from build123d import *

# Parameters (mm, degrees)
F0_R     = 6.477
F1_DEPTH = 6.35
F0_W     = 6.35
F0_H     = 25.4
F2_DEPTH = 6.35
F3_DEPTH = 6.35
F4_DEPTH = 6.35
F5_DEPTH = 6.35


with BuildPart() as f1:
    # F0 (on Top) → F1 (new body)
    with BuildSketch(Plane.XY):
        Polygon((184.15, 76.2), (-184.15, 76.2), (-184.15, 50.8), (-184.15, 25.4), (-184.15, 0), (-184.15, -25.4), (-184.15, -50.8), (-184.15, -76.2), (184.15, -76.2), (184.15, -50.8), (184.15, -25.4), (184.15, 0), (184.15, 25.4), (184.15, 50.8), align=None)
        with BuildLine():
            ThreePointArc((-157.1244, 0), (-163.6014, -6.477), (-170.0784, 0))
            ThreePointArc((-170.0784, 0), (-163.6014, 6.477), (-157.1244, 0))
        make_face(mode=Mode.SUBTRACT)
        Polygon((-88.9, -3.175), (-88.9, 0), (-88.9, 3.175), (-76.2, 3.175), (-76.2, 0), (-76.2, -3.175), align=None, mode=Mode.SUBTRACT)
        Polygon((-31.75, -3.175), (-31.75, 0), (-31.75, 3.175), (-19.05, 3.175), (-19.05, 0), (-19.05, -3.175), align=None, mode=Mode.SUBTRACT)
        Polygon((25.4, -3.175), (25.4, 0), (25.4, 3.175), (38.1, 3.175), (38.1, 0), (38.1, -3.175), align=None, mode=Mode.SUBTRACT)
        with Locations((96.52, 0)):
            Circle(F0_R, mode=Mode.SUBTRACT)
    extrude(amount=F1_DEPTH)

    # F0 (on Top) → F2 (join)
    with BuildSketch(Plane.XY):
        with Locations((187.325, -38.1)):
            Rectangle(F0_W, F0_H)
    extrude(amount=F2_DEPTH)

    # F0 (on Top) → F3 (join)
    with BuildSketch(Plane.XY):
        with Locations((187.325, 38.1)):
            Rectangle(F0_W, F0_H)
    extrude(amount=F3_DEPTH)

    # F0 (on Top) → F4 (join)
    with BuildSketch(Plane.XY):
        with Locations((-187.325, -38.1)):
            Rectangle(F0_W, F0_H)
    extrude(amount=F4_DEPTH)

    # F0 (on Top) → F5 (join)
    with BuildSketch(Plane.XY):
        with Locations((-187.325, 38.1)):
            Rectangle(F0_W, F0_H)
    extrude(amount=F5_DEPTH)


solid = f1.part
Geometry: final body of the model. Coordinates: model frame, mm. A direction names the side the tool comes from. Coordinates: 2 decimals unless noted, no trailing zeros. Order: outer loops, then holes, each group sorted by start corner. A loop starts at its lowest first (then second) coordinate and runs counter-clockwise, first axis right, second up.
(1) Access query for faces 1 (the face through (38.1, 0, 3)), 2 (the face through (-184.15, 64, 3)), 3 (the face through (187, 50.8, 3)), 4 (the face through (187, -50.8, 3)). Directions: +Z, -Z, +X, -X, +Y, -Y. A direction counts if a zero-diameter tool reaches every point of the face in a straight line with its end or side. Return the directions, or none.
(2) Section query B-B (x = 96.52). Return the cut outline in (y, z), plus the area to 3 significant figures.
(3) First-contact query: pin 1 (3 mm diameter, centred on y = -57.5, z = 3.5, fed in from -X); pin 2 (1.5 mm diameter, centred on y = 12, z = 1.5, fed in from +X); pin 3 (3 mm diameter, centred on x = 187.5, z = 3.5, fed in from +Y). Flat tips, straight axial feed; report the tip coordinate or a pass-through.
(4) Draft query along Y for faces 5 (the face through (-31.75, 0, 3)), 6 (the face through (-187, -50.8, 3)), 7 (the face through (-3, 1, 6.35)), 8 (the face through (-82, -3.175, 3)). Return one class per face: pulls with the +Y half, pulls with the -Y half, needs draft (parallel to the pull), parting line crosses it, or undercut.
(5) Section query C-C (y = -22). Return the cut outline in (x, z), plus the area to 3 significant figures.
(6) Section query A-A (z = 4.25). State how many separate pieces and enclosed holes the cut face has, plus the area to 3 significant figures.
(7) Material intervals for probe 1 along Y at (x, z) = (35, 6) (3 decimals); probe 2 along Y at (x, z) = (96.52, 1.75); probe 3 along X at (y, z) = (70, 6.25), sorted ascending.
Solution:
1. face 1: +Z, -Z
1. face 2: +Z, -Z, -X, +Y
1. face 3: +Z, -Z, +X, +Y
1. face 4: +Z, -Z, +X, -Y
2. outline: (-76.2, 0) - (-6.48, 0) - (-6.48, 6.35) - (-76.2, 6.35) - close; (6.48, 0) - (76.2, 0) - (76.2, 6.35) - (6.48, 6.35) - close
2. area: 885 mm2
3. pin 1: stops at x = -184.15
3. pin 2: stops at x = 184.15
3. pin 3: stops at y = 50.8
4. face 5: undercut
4. face 6: pulls with the -Y half
4. face 7: needs draft
4. face 8: undercut
5. outline: (-184.15, 0) - (184.15, 0) - (184.15, 6.35) - (-184.15, 6.35) - close
5. area: 2,340 mm2
6. separate pieces: 1
6. enclosed holes: 5
6. area: 56,300 mm2
7. probe 1: y = -76.2 to -3.175, 3.175 to 76.2
7. probe 2: y = -76.2 to -6.48, 6.48 to 76.2
7. probe 3: x = -184.15 to 184.15
